The listing builds one solid part. Answer for the finished solid, in the listing's coordinates (mm). Coordinates: 2 decimals unless noted, no trailing zeros. Order: outer loops, then holes, each group sorted by start corner. A loop starts at its lowest first (then second) coordinate and runs counter-clockwise, first axis right, second up.
from build123d import *

# Parameters (mm, degrees)
BASE_FLANGE1_DEPTH = 1.5
FILLET1_R          = 10
SKETCH6_R          = 2.5
CUT_EXTRUDE1_DEPTH = 10


# Sheet-metal steps are written as plain solids
with BuildPart() as part:
    # Sketch1 → Base-Flange1 (new body)
    with BuildSketch(Plane.XY):
        Polygon((116.381309109, -54.730517105), (-116.381309109, -54.730517105), (-84.350299428, -287.658470614), (84.350299428, -287.658470614), align=None)
    extrude(amount=-BASE_FLANGE1_DEPTH)

    # Fillet1
    fillet1_edges = [part.edges().sort_by_distance(p)[0] for p in [
        (84.350299428, -287.658470614, -0.75),
        (-84.350299428, -287.658470614, -0.75),
        (-116.381309109, -54.730517105, -0.75),
        (116.381309109, -54.730517105, -0.75),
    ]]
    fillet(fillet1_edges, radius=FILLET1_R)

    # Sketch6 → Cut-Extrude1 (cut)
    with BuildSketch(Plane(origin=(0, 0, -1.5), x_dir=(-1, 0, 0), z_dir=(0, 0, -1))):
        with Locations((-102.757991697, -80.676477358)):
            Circle(SKETCH6_R)
        with Locations((-90.497057702, -169.837396474)):
            Circle(SKETCH6_R)
        with Locations((-78.236123708, -258.99831559)):
            Circle(SKETCH6_R)
        with Locations((102.722754997, -80.671631795)):
            Circle(SKETCH6_R)
        with Locations((90.497057702, -169.837396474)):
            Circle(SKETCH6_R)
        with Locations((78.236123708, -258.99831559)):
            Circle(SKETCH6_R)
    extrude(amount=-CUT_EXTRUDE1_DEPTH, mode=Mode.SUBTRACT)


solid = part.part
1) Section C-C (y = -189.5) is taken. Give the vertices of the cut face in (x, z), then the cut area to 3 significant figures.
2) Section B-B (y = -140) is taken. Give the vertices of the cut face in (x, z), then the cut area to 3 significant figures.
3) Determine the mould class of faces 1 (the face through (-100.383, -171.066, -0.74)), 2 (the face through (-2, -170, -1.5)), 3 (the face through (99.973, -174.047, -0.74)), 4 (the face through (-91.84, -167.73, -0.76)) for opening direction X: released by +X, released by -X, zero draft, split by the parting line, or undercut.
4) Section A-A (z = -0.45) is taken. Give the vertices of the cut face in (x, y).
5) This flat-tipped pin is pushed along its axis until it touches: P1, Ø3, axis at x = -102.72, y = -80.67, coming from the -Z side. Where does it stop, or does it pass through?
6) Consider L1, parallel to X at y = -78.5, z = -0.15; L2, parallel to X at y = -80.5, z = -0.6; L3, parallel to X at y = -234.5, z = -0.75. Determine where each line is inside the solid, lowest interval first.
Filled sheet:
1. outline: (-97.85, -1.5) - (97.85, -1.5) - (97.85, 0) - (-97.85, 0) - close
1. area: 294 mm2
2. outline: (-104.66, -1.5) - (104.66, -1.5) - (104.66, 0) - (-104.66, 0) - close
2. area: 314 mm2
3. face 1: released by -X
3. face 2: zero draft
3. face 3: released by +X
3. face 4: undercut
4. outline: (-114.82, -66.09) - (-85.54, -279.02) arc R10 ccw to (-75.63, -287.66) - (75.63, -287.66) arc R10 ccw to (85.54, -279.02) - (114.82, -66.09) arc R10 ccw to (104.91, -54.73) - (-104.91, -54.73) arc R10 ccw to start; hole circle Ø5 at (-102.72, -80.67); hole circle Ø5 at (-90.5, -169.84); hole circle Ø5 at (-78.24, -259); hole circle Ø5 at (78.24, -259); hole circle Ø5 at (90.5, -169.84); hole circle Ø5 at (102.76, -80.68)
5. P1: passes through
6. L1: x = -113.11 to -103.96, -101.48 to 101.53, 103.99 to 113.11
6. L2: x = -112.84 to -105.22, -100.23 to 100.26, 105.25 to 112.84
6. L3: x = -91.66 to 91.66
